Autodesk Fusion 360 part; units mm, degrees
sketch "Skizze1" plane through (0, 0, 0) normal (0, 0, 1) x (1, 0, 0)
  line L0 (-22, 5) -> (22, 5)
  line L1 (22, 5) -> (22, -5)
  line L2 (22, -5) -> (-22, -5)
  line L3 (-22, -5) -> (-22, 5)
  circle A0 centre (-22, 0) radius 3.5
  circle A1 centre (22, 0) radius 3.5
  circle A2 centre (-22, 0) radius 5
  circle A3 centre (22, 0) radius 5
  line L4 (-13.5, 5) -> (13.5, 5)
  line L5 (13.5, -5) -> (-13.5, -5)
  circle A4 centre (-22, 0) radius 3
  circle A5 centre (22, 0) radius 3
  circle A6 centre (-5.06, 0) radius 1.65
  circle A7 centre (5.06, 0) radius 1.65
  line L6 (-7.71, 5) -> (7.71, 5)
  line L7 (7.71, -5) -> (-7.71, -5)
  line L8 (-7.71, 5) -> (7.71, 5)
  line L9 (7.71, 5) -> (7.71, -5)
  line L10 (7.71, -5) -> (-7.71, -5)
  line L11 (-7.71, -5) -> (-7.71, 5)
  dimension "d1" = 44
  dimension "d2" = 22
  dimension "d3" = 10
  dimension "d4" = 5
  dimension "d5" = 7
  dimension "d6" = 7
  dimension "d7" = 10
  dimension "d8" = 10
  dimension "d11" = 10
  dimension "d12" = 0
  dimension "d18" = 6
  dimension "d19" = 6
  dimension "d22" = 3.3
  dimension "d23" = 3.3
  dimension "d28" = 10
  dimension "d35" = 15.42
  dimension "d36" = 10
  dimension "d37" = 14.29
  dimension "d40" = 2.65
  dimension "d41" = 2.65
extrude "Extrusion1" add sketch "Skizze1" along normal blind 3 contours L3 A0 A2 | L0 L2 A2 L4 L5 L11 | L3 A0 A2 | L0 L2 L4 L5 L6 L7 L8 L9 L10 L11 | L0 L2 A3 L4 L5 L9 | L1 A1 A3 | L1 A1 A3
extrude "Extrusion3" add sketch "Skizze1" along normal blind 1 contours L3 A0 A4 | L3 A0 A4 | L1 A1 A5 | L1 A1 A5
extrude "Extrusion6" add sketch "Skizze1" along normal blind 18.3 from surface at 3 contours L0 L2 L4 L5 L6 L7 L8 L9 L10 L11
fillet "Abrundung1" radius 2 4 edges at (7.71, 5, 12.15) (-7.71, 5, 12.15) (-7.71, -5, 12.15) (7.71, -5, 12.15)
equation "d2 = d1 / 2"
equation "d4 = d3 / 2"
equation "d6 = d5"
equation "d7 = d3"
equation "d8 = d7"
equation "d11 = d3"
equation "d12 = ( d3 - d11 ) / 2"
equation "d18 = d5 - 1 mm"
equation "d19 = d18"
equation "d23 = d22"
equation "d24 = d31 / 2"
equation "d28 = d11"
equation "d29 = 15.22 mm + 0.2 mm"
equation "d35 = 15.22 mm + 0.2 mm"
equation "d36 = d11"
equation "d37 = ( d1 - d29 ) / 2"
equation "d40 = d41"
equation "d41 = 1.00 mm + d22 / 2"
equation "d43 = 20.3 mm - 3 mm + 1 mm"
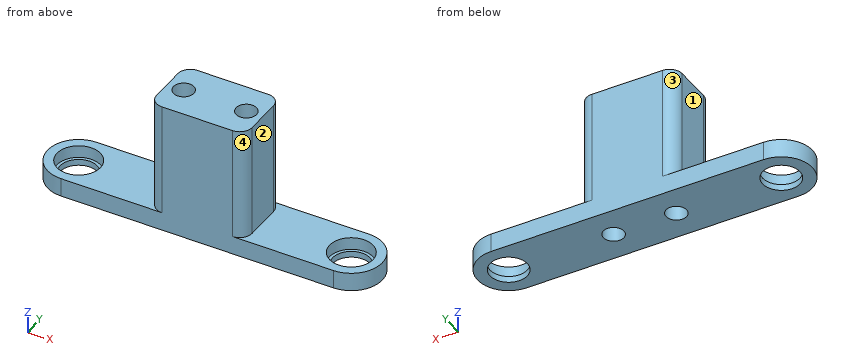
Can you work these out from the model? Positions are in its coordinate system, mm. Face numbers are marked on the shaded views. A direction names the side the tool comes from. Give positions to 0.01 mm unless a question says otherwise; leave off trailing zeros. Loops run counter-clockwise (first coordinate to the right, second up) from the corner with the lowest first, then second, coordinate; pieces in that order, holes last. Notation, with made-up numbers: M 76,71.25 L 118,71.25 A27 ccw 118,97.25 Z; hole C 3.5,-27.5 d7. An arc over 180 degrees is marked long. Answer in a Markdown table with one row per item.
1. Suppose I cut it at B-B on z = 13.5. Write out the boundary of the cut face in (x, y).
Taken from the geometry:
| item | result |
|---|---|
| outline | M -7.71,-3 A2 ccw -5.71,-5 L 5.71,-5 A2 ccw 7.71,-3 L 7.71,3 A2 ccw 5.71,5 L -5.71,5 A2 ccw -7.71,3 Z; hole C -5.06,0 d3.3; hole C 5.06,0 d3.3 |
2. Which directions (+Z, -Z, +X, -X, +Y, -Y) give clear straight access to the entire face, cutting with the end or side of a thin tool? Please do the marked faces 1, 2, 3 and 4.
Taken from the geometry:
| item | result |
|---|---|
| face 1 | +Z, -X, +Y, -Y |
| face 2 | +Z, +X, +Y, -Y |
| face 3 | +Z, -X, +Y |
| face 4 | +Z, +X, -Y |
3. If I drill on line 1 along Y through (x, z) = (-22, 0.4); line 2 along X through (y, z) = (-1.5, 12); line 3 along X through (y, z) = (-0.5, 20.75), over which ranges is the centre line in solid material (lowest first)?
Taken from the geometry:
| item | result |
|---|---|
| line 1 | y = -5 to -3, 3 to 5 |
| line 2 | x = -7.71 to -5.75, -4.37 to 4.37, 5.75 to 7.71 |
| line 3 | x = -7.71 to -6.63, -3.49 to 3.49, 6.63 to 7.71 |
4. Suppose I cut it at A-A on y = 0. Count the separate pieces of the cut face and the enclosed holes in it, plus the area to 3 significant figures.
Taken from the geometry:
| item | result |
|---|---|
| separate pieces | 5 |
| enclosed holes | 0 |
| area | 264 mm² |
5. For pin 1 Ø5.5 at (x, y) = (22, 0) entering from -Z; pin 2 Ø5 at (x, y) = (13.5, -1) entering from +Z; pin 3 Ø2 at (y, z) = (-3.5, 2.5) entering from -X; pin 4 Ø3 at (y, z) = (-0.5, 11.5) entering from -X, each with a flat end and sliding along its axis, tell me the tip position at first contact or that it passes through.
Taken from the geometry:
| item | result |
|---|---|
| pin 1 | passes through |
| pin 2 | stops at z = 3 |
| pin 3 | stops at x = -26.33 |
| pin 4 | stops at x = -7.71 |
6. Suppose I cut it at C-C on x = -5.06. Write out the boundary of the cut face in (y, z).
Taken from the geometry:
| item | result |
|---|---|
| outline | M -5,0 L -1.65,0 L -1.65,21.3 L -5,21.3 Z; M 1.65,0 L 5,0 L 5,21.3 L 1.65,21.3 Z |
7. Suppose I cut it at D-D on z = 1.75. Write out the boundary of the cut face in (x, y), plus the area to 3 significant figures.
Taken from the geometry:
| item | result |
|---|---|
| outline | M -22,-5 L 22,-5 A5 ccw 22,5 L -22,5 A5 ccw Z; hole C -22,0 d7; hole C -5.06,0 d3.3; hole C 5.06,0 d3.3; hole C 22,0 d7 |
| area | 424 mm² |
